from build123d import *

# Parameters (mm, degrees)
SKETCH_1_W          = 75
SKETCH_1_H          = 100
EXTRUDE_1_DEPTH     = 16
CUT_EXTRUDE_5_REACH = 128.02
SKETCH_8_R          = 1.45
CUT_EXTRUDE_7_DEPTH = 127.019839708
SKETCH_9_W          = 40
SKETCH_9_H          = 16
EXTRUDE_2_DEPTH     = 5
SKETCH_10_R         = 2.25
CUT_EXTRUDE_8_DEPTH = 5
CUT_EXTRUDE_START   = -5
SKETCH_11_R         = 2.25
CUT_EXTRUDE_9_DEPTH = 5


with BuildPart() as part:
    # 草图1 → 凸台-拉伸1 (new body)
    with BuildSketch(Plane(origin=(0, 0, 0), x_dir=(1, 0, 0), z_dir=(0, 1, 0))):
        with Locations((-37.5, 50)):
            Rectangle(SKETCH_1_W, SKETCH_1_H)
    extrude(amount=EXTRUDE_1_DEPTH)

    # 草图6 → 切除-拉伸5 (cut, up to next)
    with BuildSketch(Plane(origin=(0, 16, 0), x_dir=(1, 0, 0), z_dir=(0, 1, 0)), mode=Mode.PRIVATE) as cut_extrude_5_sk1:
        Polygon((-40, 45), (-5, 45), (-5, 5), (-40, 5), (-40, 25), (-70, 25), (-70, 45), align=None)
    cut_extrude_5_tool1 = extrude(cut_extrude_5_sk1.sketch, amount=-CUT_EXTRUDE_5_REACH, mode=Mode.PRIVATE) & part.part
    # 草图6 → 切除-拉伸5 (cut, up to next)
    with BuildSketch(Plane(origin=(0, 16, 0), x_dir=(1, 0, 0), z_dir=(0, 1, 0)), mode=Mode.PRIVATE) as cut_extrude_5_sk2:
        Polygon((-40, 95), (-5, 95), (-5, 55), (-40, 55), (-70, 55), (-70, 75), (-40, 75), align=None)
    cut_extrude_5_tool2 = extrude(cut_extrude_5_sk2.sketch, amount=-CUT_EXTRUDE_5_REACH, mode=Mode.PRIVATE) & part.part
    add(cut_extrude_5_tool1.solids().sort_by_distance((-32.25, 16, -28))[0], mode=Mode.SUBTRACT)
    add(cut_extrude_5_tool2.solids().sort_by_distance((-32.25, 16, -72))[0], mode=Mode.SUBTRACT)

    # 草图8 → 切除-拉伸7 (cut, through all)
    with BuildSketch(Plane(origin=(0, 16, 0), x_dir=(1, 0, 0), z_dir=(0, 1, 0))):
        with Locations(Location((-72, 97, 0), (0, 0, 270))):
            Circle(SKETCH_8_R)
        with Locations(Location((-72, 83, 0), (0, 0, 270))):
            Circle(SKETCH_8_R)
        with Locations(Location((-48, 97, 0), (0, 0, 270))):
            Circle(SKETCH_8_R)
        with Locations(Location((-48, 83, 0), (0, 0, 270))):
            Circle(SKETCH_8_R)
        with Locations(Location((-48, 17, 0), (0, 0, 90))):
            Circle(SKETCH_8_R)
        with Locations(Location((-48, 3, 0), (0, 0, 90))):
            Circle(SKETCH_8_R)
        with Locations(Location((-72, 17, 0), (0, 0, 90))):
            Circle(SKETCH_8_R)
        with Locations(Location((-72, 3, 0), (0, 0, 90))):
            Circle(SKETCH_8_R)
    extrude(amount=-CUT_EXTRUDE_7_DEPTH, mode=Mode.SUBTRACT)

    # 草图9 → 凸台-拉伸2 (add)
    with BuildSketch(Plane.ZY.offset(5)):
        with Locations((-25, 8)):
            Rectangle(SKETCH_9_W, SKETCH_9_H)
        with Locations((-75, 8)):
            Rectangle(SKETCH_9_W, SKETCH_9_H)
    extrude(amount=EXTRUDE_2_DEPTH)

    # 草图10 → 切除-拉伸8 (cut)
    with BuildSketch(Plane(origin=(0, 16, 0), x_dir=(1, 0, 0), z_dir=(0, 1, 0))):
        with Locations(Location((-5, 95, 0), (0, 0, 270))):
            Circle(SKETCH_10_R)
        with Locations(Location((-5, 5, 0), (0, 0, 90))):
            Circle(SKETCH_10_R)
    extrude(amount=-CUT_EXTRUDE_8_DEPTH, mode=Mode.SUBTRACT)

    # 草图11 → 切除-拉伸9 (cut)
    with BuildSketch(Plane.XZ.offset(CUT_EXTRUDE_START)):
        with Locations(Location((-5, -95, 0), (0, 0, 90))):
            Circle(SKETCH_11_R)
        with Locations(Location((-5, -5, 0), (0, 0, 270))):
            Circle(SKETCH_11_R)
    extrude(amount=CUT_EXTRUDE_9_DEPTH, mode=Mode.SUBTRACT)


solid = part.part
Input: part model. Units: mm. Frame: model coordinates. A direction names the side the tool comes from. Coordinates: 2 decimals unless noted, no trailing zeros. Loops run counter-clockwise (first coordinate to the right, second up) from the corner with the lowest first, then second, coordinate; pieces in that order, holes last. Notation, with made-up numbers: (-1.5, 3) -> (46.5, 3) arc R7 ccw to (46.5, 10) -> close; hole circle Ø11 at (82, 36.5). An arc over 180 degrees is marked (long way). Write item = value, one per line. Start each with the question number.
Item 1: Cut plane B-B, the plane z = -83. Return loops of the section in (x, y), plus the area to 3 significant figures.
Item 2: Material intervals for line 1 (Z direction, x = -18.5, y = 15); line 2 (X direction, y = 11, z = -83); line 3 (X direction, y = 1.25, z = -70), sorted ascending.
Item 3: Cut plane A-A, the plane x = -55. Return loops of the section in (y, z).
Item 4: Cut plane C-C, the plane x = -72. Return loops of the section in (y, z), plus the area to 3 significant figures.
Item 5: First-contact query: P1, Ø12, axis at x = -52.5, z = -35.5, coming from the +Y side. Flat tip, straight axial feed; report the tip coordinate or a pass-through.
Item 6: Mould query, pull axis X, two halves, no side actions, for faces 4 (the face through (-5, 11, -95)), 5 (the face through (-38, 8, -100)). Classes: pulls with the +X half, pulls with the -X half, needs draft (parallel to the pull), parting line crosses it, or undercut.
Item 7: Reachability of faces 1 (the face through (-40, 8, -85)), 2 (the face through (-5.676, 2.535, -92.854)), 3 (the face through (-5.676, 13.535, -7.146)) from +Z, -Z, +X, -X, +Y, -Y: full face, straight path, thin tool, end or side. Return the list, or none.
Item 8: Cut plane D-D, the plane y = 6.75. Count the separate pieces of the cut face and the enclosed holes in it, plus the area to 3 significant figures.
Ans:
q1.outline = (-75, 0) -> (-73.45, 0) -> (-73.45, 16) -> (-75, 16) -> close; (-70.55, 0) -> (-49.45, 0) -> (-49.45, 16) -> (-70.55, 16) -> close; (-46.55, 0) -> (-40, 0) -> (-40, 16) -> (-46.55, 16) -> close; (-10, 0) -> (0, 0) -> (0, 16) -> (-10, 16) -> close
q1.area = 627 mm²
q2.line_1 = -100 to -95, -55 to -45, -5 to 0
q2.line_2 = -75 to -73.45, -70.55 to -49.45, -46.55 to -40, -10 to 0
q2.line_3 = -75 to -70, -10 to 0
q3.outline = (0, -100) -> (16, -100) -> (16, -75) -> (0, -75) -> close; (0, -55) -> (16, -55) -> (16, -45) -> (0, -45) -> close; (0, -25) -> (16, -25) -> (16, 0) -> (0, 0) -> close
q4.outline = (0, -100) -> (16, -100) -> (16, -98.45) -> (0, -98.45) -> close; (0, -95.55) -> (16, -95.55) -> (16, -84.45) -> (0, -84.45) -> close; (0, -81.55) -> (16, -81.55) -> (16, -18.45) -> (0, -18.45) -> close; (0, -15.55) -> (16, -15.55) -> (16, -4.45) -> (0, -4.45) -> close; (0, -1.55) -> (16, -1.55) -> (16, 0) -> (0, 0) -> close
q4.area = 1,410 mm²
q5.P1 = through
q6.face_4 = undercut
q6.face_5 = needs draft
q7.face_1 = +Y, -Y
q7.face_2 = -Y
q7.face_3 = +Y
q8.separate_pieces = 1
q8.enclosed_holes = 10
q8.area = 3,850 mm²
